The model under review builds one solid part; all positions refer to its coordinate system, in mm. Face numbers are marked on the shaded views. A direction names the side the tool comes from. Round coordinates to 2 decimals unless told otherwise and drop trailing zeros. Order: outer loops, then holes, each group sorted by start corner. A loop starts at its lowest first (then second) coordinate and runs counter-clockwise, first axis right, second up. Notation, with made-up numbers: M 15.25,8 L 56.25,8 A30 ccw 56.25,40 Z; hole C 54.5,-1 d10. An arc over 180 degrees is marked long. Answer as CSV lines item,"result". Start each with the question number.
from build123d import *

# Parameters (mm, degrees)
M2X0_4_TAPPED_HOLE1_D = 1.6


with BuildPart() as part:
    # Sketch1 → Revolve1 (revolve)
    with BuildSketch(Plane(origin=(0, 0, 0), x_dir=(-1, 0, 0), z_dir=(0, 0, -1)), mode=Mode.PRIVATE) as revolve1_sk:
        with BuildLine():
            Line((50, 2.1), (50, 3))
            add(Edge.make_bspline(
                [(49, 4), (49.333333333, 3.666666667), (49.666666667, 3.333333333), (50, 3)],
                knots=[0, 0, 0, 0, 1, 1, 1, 1], degree=3))
            Line((49, 4), (36.9, 4))
            Line((36.9, 4), (36.9, 3.8))
            Line((36.9, 3.8), (36, 3.8))
            Line((36, 3.8), (36, 4))
            Line((36, 4), (7.2, 4))
            ThreePointArc((7.2, 4), (7.058578644, 4.058578644), (7, 4.2))
            Line((7, 4.2), (7, 6))
            Line((7, 6), (0, 6))
            Line((0, 6), (0, 10))
            Line((0, 10), (-2.5, 10))
            Line((-2.5, 10), (-2.5, 2.1))
            Line((-2.5, 2.1), (50, 2.1))
        make_face()
    revolve(revolve1_sk.sketch.rotate(Axis((0, 0, 0), (-1, 0, 0)), 270), axis=Axis((0, 0, 0), (-1, 0, 0)))

    # M2x0.4 Tapped Hole1 (through all)
    with Locations(Plane(origin=(2.5, 0, 0), x_dir=(0, 0, -1), z_dir=(1, 0, 0))):
        with Locations((8.5, 0), (-4.25, 7.361215932), (-4.25, -7.361215932)):
            Hole(M2X0_4_TAPPED_HOLE1_D / 2)


solid = part.part
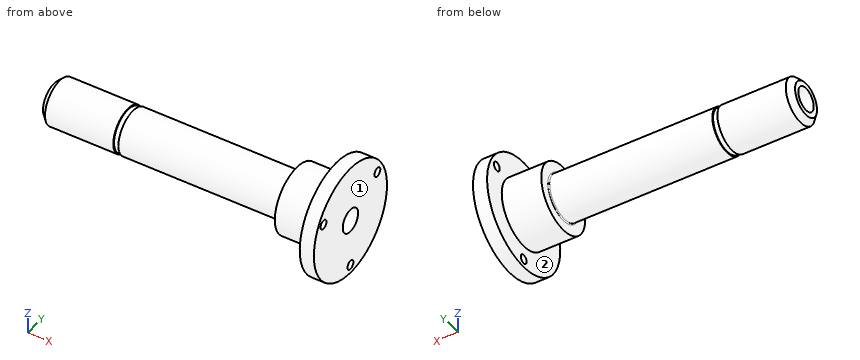
Item 1: For pin 1 (2 mm diameter, centred on x = -9, y = 0, fed in from -Z); pin 2 (1.8 mm diameter, centred on y = -7.36, z = 4.25, fed in from -X); pin 3 (1.5 mm diameter, centred on x = -25.5, z = 3.5, fed in from -Y); pin 4 (1.5 mm diameter, centred on y = 1, z = -0.5, fed in from -X), all flat-tipped, find the tip position at first contact; note any pin that passes through.
Item 2: Wall thickness on probe 1 along Y at (x, z) = (1.75, 4.25); probe 2 along X at (y, z) = (-3.5, 6); probe 3 along X at (y, z) = (0.25, 4.25): over which ranges is each line inside the solid? List them lowest first. Write a range as [from, to].
Item 3: Consider section C-C (x = -10). State the section outline as (y, z) points.
Item 4: Consider section A-A (z = -8.5). State the section outline as (x, y) points, and give its area (3 significant figures).
Item 5: Tool access review of the marked faces 1 and 2: name each direction out of +Z, -Z, +X, -X, +Y, -Y from which nothing blocks a thin tool from reaching the whole face with its end or side.
Item 6: Consider section B-B (y = 0). State how many separate pieces and enclosed holes the cut face has, and give its area (3 significant figures).
Reported:
1,pin 1,"stops at z = -4"
1,pin 2,"stops at x = 0"
1,pin 3,"stops at y = -2.9"
1,pin 4,"passes through"
2,probe 1,"y = [-9.05, -8.16], [-6.56, 6.56], [8.16, 9.05]"
2,probe 2,"x = [0, 2.5]"
2,probe 3,"x = [-7, 2.5]"
3,outline,"C 0,0 d8; hole C 0,0 d4.2"
4,outline,"M 0,-5.27 L 2.5,-5.27 L 2.5,-0.8 L 0,-0.8 Z; M 0,0.8 L 2.5,0.8 L 2.5,5.27 L 0,5.27 Z"
4,area,"22.3 mm²"
5,face 1,"+Z, -Z, +X, +Y, -Y"
5,face 2,"-X"
6,separate pieces,"3"
6,enclosed holes,"0"
6,area,"252 mm²"
